Here's how the part is built. I have some questions about the finished solid (model axes, mm). Coordinates: 2 decimals unless noted, no trailing zeros. Write each loop counter-clockwise with the first axis right and the second up, starting at its lowest first coordinate (ties: lowest second). Pieces come first, ordered by that corner, then holes. Notation, with made-up numbers: (77, 0) - (88, 0) arc R27 cw to (88, 16) - close; hole circle Ø7 at (-19, 27.25). An arc over 180 degrees is marked (long way). Answer in a Markdown table with one row per item. Add a question column.
Item 1: If I drill on probe 1 along X at (y, z) = (-0.6, 3); probe 2 along Z at (x, y) = (-50.5, -2.2); probe 3 along X at (y, z) = (-3.25, 4), over which ranges is the centre line in solid material (lowest first)? Write a range as from..to.
Item 2: I'm going to push flat-ended pins straight in: pin 1 (2 mm diameter, centred on x = 50, y = -2.5, fed in from -Z); pin 2 (2.5 mm diameter, centred on x = 31, y = -3.5, fed in from -Z); pin 3 (0.5 mm diameter, centred on x = 26.5, z = 6.5, fed in from -Y); pin 4 (0.8 mm diameter, centred on x = -22, y = -3.5, fed in from +Z). Where does each tip first touch, or does it pass through?
Item 3: Imagine slicing it at A-A (x = 9). Please give me the cut outline in (y, z).
Item 4: Imagine slicing it at B-B (x = 61). Please give me the cut outline in (y, z), plus the area to 3 significant figures.
from build123d import *

# Parameters (mm, degrees)
F1_DEPTH = 5
F0_W     = 128.6
F0_H     = 1.6
F2_DEPTH = 2.5
F3_W     = 2
F3_H     = 2
F4_DEPTH = 2
F5_W     = 2
F5_H     = 2
F6_DEPTH = 2


with BuildPart() as f1:
    # F0 (on Front) → F1 (new body)
    with BuildSketch(Plane.XZ):
        Polygon((64.3, 0.177778), (64.3, 5.477778), (-64.3, 5.477778), (-64.3, 0.177778), (-36.75, 0.177778), (-36.75, 3.177778), (-23.25, 3.177778), (-23.25, 0.177778), (-16.75, 0.177778), (-16.75, 3.177778), (-3.25, 3.177778), (-3.25, 0.177778), (3.25, 0.177778), (3.25, 3.177778), (16.75, 3.177778), (16.75, 0.177778), (23.25, 0.177778), (23.25, 3.177778), (36.75, 3.177778), (36.75, 0.177778), align=None)
    extrude(amount=F1_DEPTH)

    # F0 (on Front) → F2 (join)
    with BuildSketch(Plane.XZ):
        with BuildLine():
            Line((-64.3, 0.177778), (-64.3, 5.477778))
            ThreePointArc((-64.3, 5.477778), (-65.3, 4.477778), (-66.3, 5.477778))
            Line((-66.3, 5.477778), (-70.25, 5.477778))
            Line((-70.25, 5.477778), (-70.25, 0.177778))
            Line((-70.25, 0.177778), (-64.3, 0.177778))
        make_face()
        with Locations((0, 6.277778)):
            Rectangle(F0_W, F0_H)
        with BuildLine():
            ThreePointArc((66.3, 5.477778), (65.3, 4.477778), (64.3, 5.477778))
            Line((64.3, 5.477778), (64.3, 0.177778))
            Line((64.3, 0.177778), (70.25, 0.177778))
            Line((70.25, 0.177778), (70.25, 5.477778))
            Line((70.25, 5.477778), (66.3, 5.477778))
        make_face()
    extrude(amount=F2_DEPTH)

    # F3 (on face) → F4 (cut)
    with BuildSketch(Plane(origin=(0, 0, 0.177778), x_dir=(1, 0, 0), z_dir=(0, 0, -1))):
        with Locations((50.525, 2.5)):
            Rectangle(F3_W, F3_H)
    extrude(amount=-F4_DEPTH, mode=Mode.SUBTRACT)

    # F5 (on face) → F6 (cut)
    with BuildSketch(Plane(origin=(0, 0, 0.177778), x_dir=(1, 0, 0), z_dir=(0, 0, -1))):
        with Locations((-50.525, 2.5)):
            Rectangle(F5_W, F5_H)
    extrude(amount=-F6_DEPTH, mode=Mode.SUBTRACT)


solid = f1.part
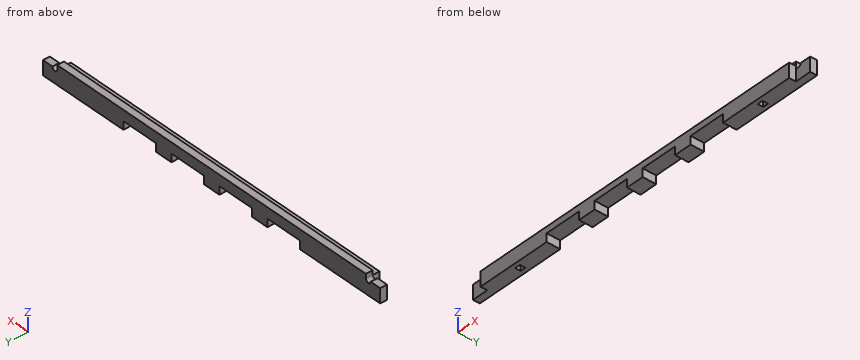
Here are the results:
| question | item | result |
|---|---|---|
| 1 | probe 1 | x = -70.25..-36.75, -23.25..-16.75, -3.25..3.25, 16.75..23.25, 36.75..70.25 |
| 1 | probe 2 | z = 2.18..7.08 |
| 1 | probe 3 | x = -64.3..64.3 |
| 2 | pin 1 | stops at z = 0.18 |
| 2 | pin 2 | stops at z = 3.18 |
| 2 | pin 3 | stops at y = -2.5 |
| 2 | pin 4 | stops at z = 5.48 |
| 3 | outline | (-5, 3.18) - (0, 3.18) - (0, 7.08) - (-2.5, 7.08) - (-2.5, 5.48) - (-5, 5.48) - close |
| 4 | outline | (-5, 0.18) - (0, 0.18) - (0, 7.08) - (-2.5, 7.08) - (-2.5, 5.48) - (-5, 5.48) - close |
| 4 | area | 30.5 mm2 |
